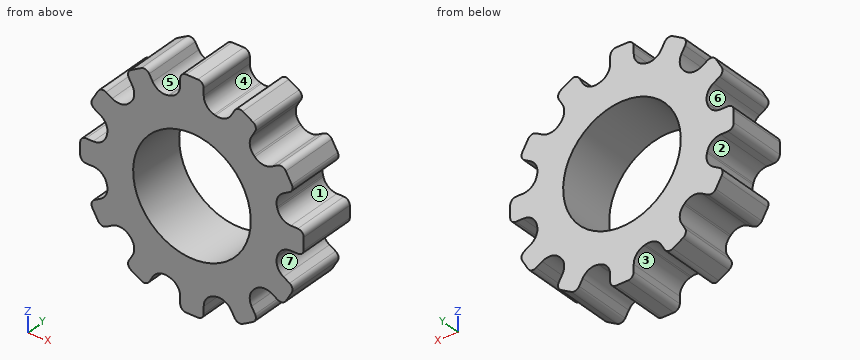
```python
from build123d import *

# Parameters (mm, degrees)
SKETCH1_R           = 6.35
BOSS_EXTRUDE1_DEPTH = 6.35


with BuildPart() as part:
    # Sketch1 → Boss-Extrude1 (new body)
    with BuildSketch(Plane(origin=(0, 0, 0), x_dir=(1, 0, 0), z_dir=(0, 1, 0))):
        with BuildLine():
            Line((-1.27, 10.670267616), (-1.27, 11.43))
            ThreePointArc((-1.27, 11.43), (-1.084012806, 11.879012806), (-0.635, 12.065))
            Line((-0.635, 12.065), (0.635, 12.065))
            ThreePointArc((0.635, 12.065), (1.084012806, 11.879012806), (1.27, 11.43))
            Line((1.27, 11.43), (1.27, 10.670267616))
            ThreePointArc((1.27, 10.670267616), (1.583306834, 9.753271395), (2.392223502, 9.219701281))
            Line((2.392223502, 9.219701281), (2.538124316, 9.180607276))
            ThreePointArc((2.538124316, 9.180607276), (3.505451757, 9.238234215), (4.235281545, 9.875722821))
            Line((4.235281545, 9.875722821), (4.615147737, 10.533670365))
            ThreePointArc((4.615147737, 10.533670365), (5.000723775, 10.829533265), (5.482573869, 10.766096497))
            Line((5.482573869, 10.766096497), (6.582426131, 10.131096497))
            ThreePointArc((6.582426131, 10.131096497), (6.878289031, 9.745520459), (6.814852263, 9.263670365))
            Line((6.814852263, 9.263670365), (6.434986071, 8.605722821))
            ThreePointArc((6.434986071, 8.605722821), (6.247819637, 7.654927381), (6.681576965, 6.788383774))
            Line((6.681576965, 6.788383774), (6.788383774, 6.681576965))
            ThreePointArc((6.788383774, 6.681576965), (7.654927381, 6.247819637), (8.605722821, 6.434986071))
            Line((8.605722821, 6.434986071), (9.263670365, 6.814852263))
            ThreePointArc((9.263670365, 6.814852263), (9.745520459, 6.878289031), (10.131096497, 6.582426131))
            Line((10.131096497, 6.582426131), (10.766096497, 5.482573869))
            ThreePointArc((10.766096497, 5.482573869), (10.829533265, 5.000723775), (10.533670365, 4.615147737))
            Line((10.533670365, 4.615147737), (9.875722821, 4.235281545))
            ThreePointArc((9.875722821, 4.235281545), (9.238234215, 3.505451757), (9.180607276, 2.538124316))
            Line((9.180607276, 2.538124316), (9.219701281, 2.392223502))
            ThreePointArc((9.219701281, 2.392223502), (9.753271395, 1.583306834), (10.670267616, 1.27))
            Line((10.670267616, 1.27), (11.43, 1.27))
            ThreePointArc((11.43, 1.27), (11.879012806, 1.084012806), (12.065, 0.635))
            Line((12.065, 0.635), (12.065, -0.635))
            ThreePointArc((12.065, -0.635), (11.879012806, -1.084012806), (11.43, -1.27))
            Line((11.43, -1.27), (10.670267616, -1.27))
            ThreePointArc((10.670267616, -1.27), (9.753271395, -1.583306834), (9.219701281, -2.392223502))
            Line((9.219701281, -2.392223502), (9.180607276, -2.538124316))
            ThreePointArc((9.180607276, -2.538124316), (9.238234215, -3.505451757), (9.875722821, -4.235281545))
            Line((9.875722821, -4.235281545), (10.533670365, -4.615147737))
            ThreePointArc((10.533670365, -4.615147737), (10.829533265, -5.000723775), (10.766096497, -5.482573869))
            Line((10.766096497, -5.482573869), (10.131096497, -6.582426131))
            ThreePointArc((10.131096497, -6.582426131), (9.745520459, -6.878289031), (9.263670365, -6.814852263))
            Line((9.263670365, -6.814852263), (8.605722821, -6.434986071))
            ThreePointArc((8.605722821, -6.434986071), (7.654927381, -6.247819637), (6.788383774, -6.681576965))
            Line((6.788383774, -6.681576965), (6.681576965, -6.788383774))
            ThreePointArc((6.681576965, -6.788383774), (6.247819637, -7.654927381), (6.434986071, -8.605722821))
            Line((6.434986071, -8.605722821), (6.814852263, -9.263670365))
            ThreePointArc((6.814852263, -9.263670365), (6.878289031, -9.745520459), (6.582426131, -10.131096497))
            Line((6.582426131, -10.131096497), (5.482573869, -10.766096497))
            ThreePointArc((5.482573869, -10.766096497), (5.000723775, -10.829533265), (4.615147737, -10.533670365))
            Line((4.615147737, -10.533670365), (4.235281545, -9.875722821))
            ThreePointArc((4.235281545, -9.875722821), (3.505451757, -9.238234215), (2.538124316, -9.180607276))
            Line((2.538124316, -9.180607276), (2.392223502, -9.219701281))
            ThreePointArc((2.392223502, -9.219701281), (1.583306834, -9.753271395), (1.27, -10.670267616))
            Line((1.27, -10.670267616), (1.27, -11.43))
            ThreePointArc((1.27, -11.43), (1.084012806, -11.879012806), (0.635, -12.065))
            Line((0.635, -12.065), (-0.635, -12.065))
            ThreePointArc((-0.635, -12.065), (-1.084012806, -11.879012806), (-1.27, -11.43))
            Line((-1.27, -11.43), (-1.27, -10.670267616))
            ThreePointArc((-1.27, -10.670267616), (-1.583306834, -9.753271395), (-2.392223502, -9.219701281))
            Line((-2.392223502, -9.219701281), (-2.538124316, -9.180607276))
            ThreePointArc((-2.538124316, -9.180607276), (-3.505451757, -9.238234215), (-4.235281545, -9.875722821))
            Line((-4.235281545, -9.875722821), (-4.615147737, -10.533670365))
            ThreePointArc((-4.615147737, -10.533670365), (-5.000723775, -10.829533265), (-5.482573869, -10.766096497))
            Line((-5.482573869, -10.766096497), (-6.582426131, -10.131096497))
            ThreePointArc((-6.582426131, -10.131096497), (-6.878289031, -9.745520459), (-6.814852263, -9.263670365))
            Line((-6.814852263, -9.263670365), (-6.434986071, -8.605722821))
            ThreePointArc((-6.434986071, -8.605722821), (-6.247819637, -7.654927381), (-6.681576965, -6.788383774))
            Line((-6.681576965, -6.788383774), (-6.788383774, -6.681576965))
            ThreePointArc((-6.788383774, -6.681576965), (-7.654927381, -6.247819637), (-8.605722821, -6.434986071))
            Line((-8.605722821, -6.434986071), (-9.263670365, -6.814852263))
            ThreePointArc((-9.263670365, -6.814852263), (-9.745520459, -6.878289031), (-10.131096497, -6.582426131))
            Line((-10.131096497, -6.582426131), (-10.766096497, -5.482573869))
            ThreePointArc((-10.766096497, -5.482573869), (-10.829533265, -5.000723775), (-10.533670365, -4.615147737))
            Line((-10.533670365, -4.615147737), (-9.875722821, -4.235281545))
            ThreePointArc((-9.875722821, -4.235281545), (-9.238234215, -3.505451757), (-9.180607276, -2.538124316))
            Line((-9.180607276, -2.538124316), (-9.219701281, -2.392223502))
            ThreePointArc((-9.219701281, -2.392223502), (-9.753271395, -1.583306834), (-10.670267616, -1.27))
            Line((-10.670267616, -1.27), (-11.43, -1.27))
            ThreePointArc((-11.43, -1.27), (-11.879012806, -1.084012806), (-12.065, -0.635))
            Line((-12.065, -0.635), (-12.065, 0.635))
            ThreePointArc((-12.065, 0.635), (-11.879012806, 1.084012806), (-11.43, 1.27))
            Line((-11.43, 1.27), (-10.670267616, 1.27))
            ThreePointArc((-10.670267616, 1.27), (-9.753271395, 1.583306834), (-9.219701281, 2.392223502))
            Line((-9.219701281, 2.392223502), (-9.180607276, 2.538124316))
            ThreePointArc((-9.180607276, 2.538124316), (-9.238234215, 3.505451757), (-9.875722821, 4.235281545))
            Line((-9.875722821, 4.235281545), (-10.533670365, 4.615147737))
            ThreePointArc((-10.533670365, 4.615147737), (-10.829533265, 5.000723775), (-10.766096497, 5.482573869))
            Line((-10.766096497, 5.482573869), (-10.131096497, 6.582426131))
            ThreePointArc((-10.131096497, 6.582426131), (-9.745520459, 6.878289031), (-9.263670365, 6.814852263))
            Line((-9.263670365, 6.814852263), (-8.605722821, 6.434986071))
            ThreePointArc((-8.605722821, 6.434986071), (-7.654927381, 6.247819637), (-6.788383774, 6.681576965))
            Line((-6.788383774, 6.681576965), (-6.681576965, 6.788383774))
            ThreePointArc((-6.681576965, 6.788383774), (-6.247819637, 7.654927381), (-6.434986071, 8.605722821))
            Line((-6.434986071, 8.605722821), (-6.814852263, 9.263670365))
            ThreePointArc((-6.814852263, 9.263670365), (-6.878289031, 9.745520459), (-6.582426131, 10.131096497))
            Line((-6.582426131, 10.131096497), (-5.482573869, 10.766096497))
            ThreePointArc((-5.482573869, 10.766096497), (-5.000723775, 10.829533265), (-4.615147737, 10.533670365))
            Line((-4.615147737, 10.533670365), (-4.235281545, 9.875722821))
            ThreePointArc((-4.235281545, 9.875722821), (-3.505451757, 9.238234215), (-2.538124316, 9.180607276))
            Line((-2.538124316, 9.180607276), (-2.392223502, 9.219701281))
            ThreePointArc((-2.392223502, 9.219701281), (-1.583306834, 9.753271395), (-1.27, 10.670267616))
        make_face()
        with Locations(Location((0, 0, 0), (0, 0, 270))):
            Circle(SKETCH1_R, mode=Mode.SUBTRACT)
    extrude(amount=BOSS_EXTRUDE1_DEPTH)


solid = part.part
```
Input: part model. Units: mm. Frame: model coordinates. Face numbers are marked on the shaded views. A direction names the side the tool comes from. Give positions to 0.01 mm unless a question says otherwise; leave off trailing zeros. Order: outer loops, then holes, each group sorted by start corner. A loop starts at its lowest first (then second) coordinate and runs counter-clockwise, first axis right, second up. Notation, with made-up numbers: M -36.5,-29.75 L 18.5,-29.75 A16 cw 18.5,-8.75 Z; hole C -25.75,69.5 d8. An arc over 180 degrees is marked long. Return JSON: item names as keys, results as strings.
1) Mould query, pull axis X, two halves, no side actions, for the marked faces 5, 6 and 7. Classes: released by +X, released by -X, zero draft, split by the parting line, or undercut.
Taken from the geometry:
{"face 5": "undercut", "face 6": "released by -X", "face 7": "released by +X"}
2) Line query: L1, parallel to X at y = 4.5, z = 0 (3 decimals); L2, parallel to Z at x = 0.25, y = 0.75 (3 decimals); L3, parallel to Z at x = -9.5, y = 2.5. Output: solid intervals per line, ascending. Write a range as [from, to].
Taken from the geometry:
{"L1": "x = [-12.065, -6.35], [6.35, 12.065]", "L2": "z = [-12.065, -6.345], [6.345, 12.065]", "L3": "z = [-6.89, -3.93], [-1.83, 1.83], [3.93, 6.89]"}
3) Access query for the marked faces 1, 2, 3 and 4. Directions: +Z, -Z, +X, -X, +Y, -Y. A direction counts if a zero-diameter tool reaches every point of the face in a straight line with its end or side. Return the directions, or none.
Taken from the geometry:
{"face 1": "+X, +Y, -Y", "face 2": "-X, +Y, -Y", "face 3": "-Z, +Y, -Y", "face 4": "+Z, +Y, -Y"}
4) Section query B-B on z = 0. Output: boundary loops of the cut face in (x, y) (3 decimals), and give its area (3 significant figures).
Taken from the geometry:
{"outline": "M -12.065,0 L -6.35,0 L -6.35,6.35 L -12.065,6.35 Z; M 6.35,0 L 12.065,0 L 12.065,6.35 L 6.35,6.35 Z", "area": "72.6 mm2"}
5) Section query A-A on x = 0. Output: boundary loops of the cut face in (y, z) (3 decimals).
Taken from the geometry:
{"outline": "M 0,-12.065 L 6.35,-12.065 L 6.35,-6.35 L 0,-6.35 Z; M 0,6.35 L 6.35,6.35 L 6.35,12.065 L 0,12.065 Z"}
6) Contact query for flat-ended pins moving along their axis: pin 1 (0.8 mm diameter, centred on y = 2.5, z = -11, fed in from +X); pin 2 (0.6 mm diameter, centred on x = -11, y = 4.5, fed in from +Z); pin 3 (1.5 mm diameter, centred on x = -3.5, y = 4, fed in from -Z). Output: stop coordinate, or through.
Taken from the geometry:
{"pin 1": "stops at x = 5.77", "pin 2": "stops at z = 5.6", "pin 3": "stops at z = -9.9"}
